The listing builds one solid part. Answer for the finished solid, in the listing's coordinates (mm). Face numbers are marked on the shaded views. A direction names the side the tool comes from. Round coordinates to 2 decimals unless told otherwise and drop trailing zeros. Write each loop counter-clockwise with the first axis right and the second up, starting at its lowest first coordinate (ties: lowest second). Pieces come first, ordered by that corner, then holes.
from build123d import *

# Parameters (mm, degrees)
SKETCH1_W      = 14
SKETCH1_H      = 18
EXTRUDE1_DEPTH = 5
SKETCH2_R      = 4
EXTRUDE2_DEPTH = 5
SKETCH3_R      = 2.1
EXTRUDE3_DEPTH = 6
EXTRUDE5_DEPTH = 5
FILLET1_R      = 3


with BuildPart() as part:
    # Sketch1 → Extrude1 (new body)
    with BuildSketch(Plane.XY):
        Rectangle(SKETCH1_W, SKETCH1_H)
    extrude(amount=EXTRUDE1_DEPTH)

    # Sketch2 → Extrude2 (add)
    with BuildSketch(Plane.XY.offset(5)):
        Circle(SKETCH2_R)
    extrude(amount=EXTRUDE2_DEPTH)

    # Sketch3 → Extrude3 (cut)
    with BuildSketch(Plane.XY.offset(10)):
        Circle(SKETCH3_R)
    extrude(amount=-EXTRUDE3_DEPTH, mode=Mode.SUBTRACT)

    # Sketch4 → Extrude5 (add)
    with BuildSketch(Plane.XY):
        Polygon((-7, 1.348977854), (-12, 1.348977854), (-12, -12), (0, -12), (0, -9), (-7, -9), align=None)
    extrude(amount=EXTRUDE5_DEPTH)

    # Fillet1
    fillet1_edges = [part.edges().sort_by_distance(p)[0] for p in [
        (0, -9, 2.5),
        (7, -9, 2.5),
        (-7, 1.348977854, 2.5),
    ]]
    fillet(fillet1_edges, radius=FILLET1_R - 0.0001)  # a hair under: the kernel refuses the full size


solid = part.part
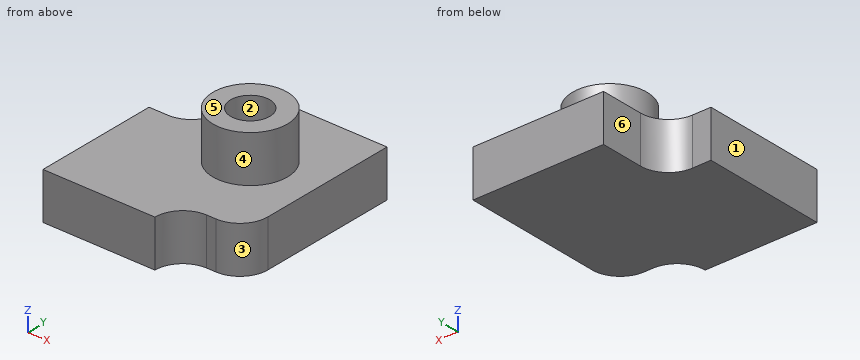
1. For a pull along X with two mould halves and no side action, classify the marked faces 1, 2 and 3 as released by +X, released by -X, zero draft, split by the parting line, or undercut.
Geometry says:
face 1: released by -X
face 2: undercut
face 3: released by +X
2. Given pin 1 (4 mm diameter, centred on x = 0, y = 0, fed in from -Z); pin 2 (1.1 mm diameter, centred on x = 3.5, z = 3.5, fed in from -Y); pin 3 (8 mm diameter, centred on x = -5.5, y = -9, fed in from +Z); pin 4 (2 mm diameter, centred on x = -2, z = 7.5, fed in from -Y), each flat-ended and moving along its own axis, determine where each tip first touches the part or whether it passes through.
Geometry says:
pin 1: stops at z = 0
pin 2: stops at y = -9
pin 3: stops at z = 5
pin 4: stops at y = -3.87
3. Straight lines are drawn through the part: line 1 along Y through (x, z) = (0, 8.75); line 2 along Z through (x, y) = (-2, -7.5); line 3 along X through (y, z) = (7, 4.75). For each, find the intervals that lie inside material, in ascending order.
Geometry says:
line 1: y = -4 to -2.1, 2.1 to 4
line 2: z = 0 to 5
line 3: x = -7 to 7
4. A tool of negligible diameter and unlimited length cuts with its end or side. For the marked faces 4, 5 and 6, from which of +Z, -Z, +X, -X, +Y, -Y can it reach the whole face along a straight path? Write none if from no direction.
Geometry says:
face 4: +Z
face 5: +Z, +X, -X, +Y, -Y
face 6: +Z, -Z, -X, +Y
5. Section B-B on y = 0 is taken. Determine the outline of the cut face in (x, z).
Geometry says:
outline: (-12, 0) - (7, 0) - (7, 5) - (4, 5) - (4, 10) - (2.1, 10) - (2.1, 4) - (-2.1, 4) - (-2.1, 10) - (-4, 10) - (-4, 5) - (-12, 5) - close
6. Section C-C on x = -10.5 is taken. Determine the outline of the cut face in (y, z).
Geometry says:
outline: (-12, 0) - (1.35, 0) - (1.35, 5) - (-12, 5) - close
